Source: three-view drawing plus pictorial views. Frame: mm from the lowest corner of the part. Coordinates: 2 decimals unless noted, no trailing zeros. Loops run counter-clockwise (first coordinate to the right, second up) from the corner with the lowest first, then second, coordinate; pieces in that order, holes last.
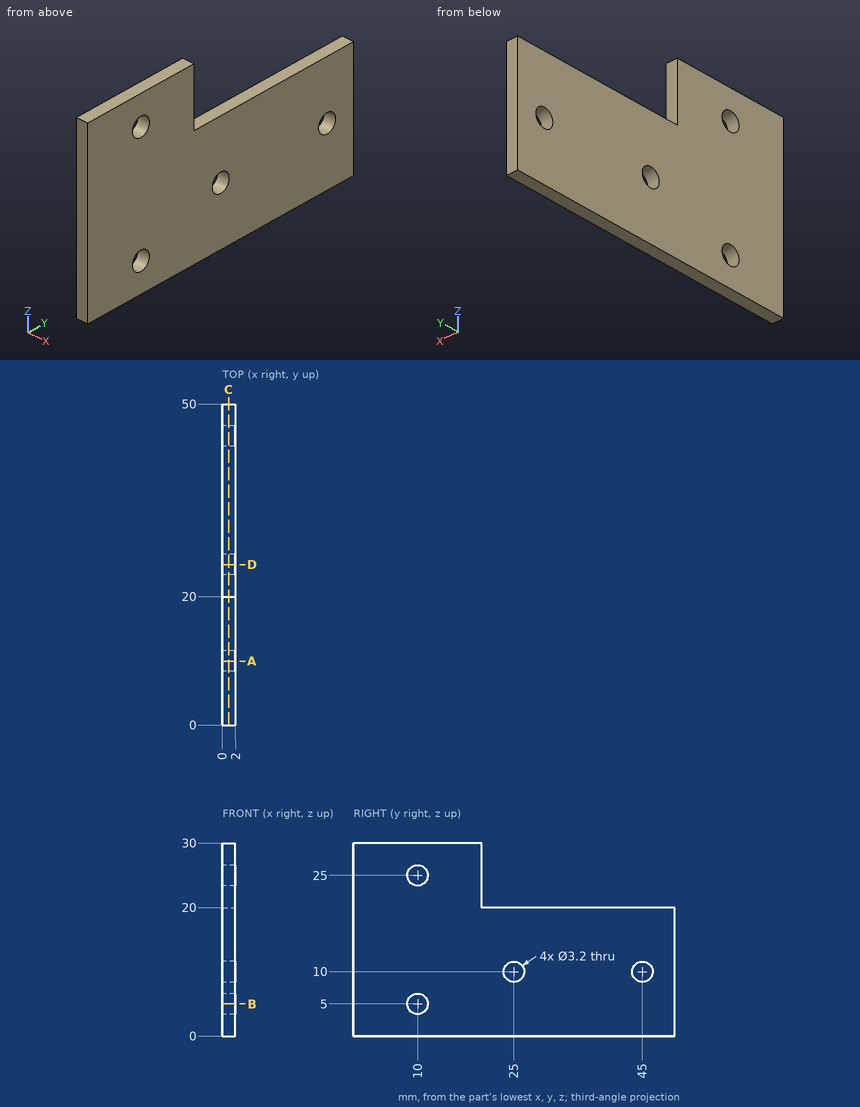
Q1. Section query C-C on x = 0.95. Return the cut outline in (y, z), then the cut area to 3 significant figures.
Q2. Section query D-D on y = 25. Return the cut outline in (x, z), then the cut area to 3 significant figures.
Q3. Section query B-B on z = 5. Return the cut outline in (x, y).
Q4. Section query A-A on y = 10. Return the cut outline in (x, z).
Q5. Material intervals for line 1 along Z through (x, y) = (1.4, 10); line 2 along Z through (x, y) = (0.8, 45); line 3 along Y through (x, z) = (1, 5), sorted ascending.
Resolved:
1. outline: (0, 0) - (50, 0) - (50, 20) - (20, 20) - (20, 30) - (0, 30) - close; hole circle Ø3.2 at (10, 5); hole circle Ø3.2 at (10, 25); hole circle Ø3.2 at (25, 10); hole circle Ø3.2 at (45, 10)
1. area: 1,170 mm2
2. outline: (0, 0) - (2, 0) - (2, 8.4) - (0, 8.4) - close; (0, 11.6) - (2, 11.6) - (2, 20) - (0, 20) - close
2. area: 33.6 mm2
3. outline: (0, 0) - (2, 0) - (2, 8.4) - (0, 8.4) - close; (0, 11.6) - (2, 11.6) - (2, 50) - (0, 50) - close
4. outline: (0, 0) - (2, 0) - (2, 3.4) - (0, 3.4) - close; (0, 6.6) - (2, 6.6) - (2, 23.4) - (0, 23.4) - close; (0, 26.6) - (2, 26.6) - (2, 30) - (0, 30) - close
5. line 1: z = 0 to 3.4, 6.6 to 23.4, 26.6 to 30
5. line 2: z = 0 to 8.4, 11.6 to 20
5. line 3: y = 0 to 8.4, 11.6 to 50
